```python
from build123d import *

# Parameters (mm, degrees)
SKETCH_R          = 5
PAD_DEPTH         = 5
POCKET_DEPTH      = 25.001
POCKET_DEPTH_BACK = 25.001


with BuildPart() as part:
    # Sketch → Pad (new body)
    with BuildSketch(Plane.XY):
        with BuildLine():
            Line((-50, 15), (-50, -15))
            ThreePointArc((-50, -15), (-47.071068, -22.071068), (-40, -25))
            Line((-40, -25), (0, -25))
            Line((0, -25), (0, 25))
            Line((0, 25), (-40, 25))
            ThreePointArc((-40, 25), (-47.071068, 22.071068), (-50, 15))
        make_face()
        with Locations((-40, 15)):
            Circle(SKETCH_R, mode=Mode.SUBTRACT)
        with Locations((-40, -15)):
            Circle(SKETCH_R, mode=Mode.SUBTRACT)
    extrude(amount=PAD_DEPTH)

    # Sketch001 → Pocket (cut, two sides)
    with BuildSketch(Plane.XZ) as pocket_sk:
        Polygon((0, 3), (-24, 3), (-24.890457, 5), (0, 5), align=None)
    extrude(amount=-POCKET_DEPTH, mode=Mode.SUBTRACT)
    extrude(pocket_sk.sketch, amount=POCKET_DEPTH_BACK, mode=Mode.SUBTRACT)

    # Mirrored: part across YZ


with BuildPart() as part_1:
    add(part.part)
    add(part.part.mirror(Plane.YZ))


solid = part_1.part
```
Verification items for the finished model (mm, model axes). A direction names the side the tool comes from. Round coordinates to 2 decimals unless told otherwise and drop trailing zeros. Order: outer loops, then holes, each group sorted by start corner. A loop starts at its lowest first (then second) coordinate and runs counter-clockwise, first axis right, second up.
1) Cross-section at D-D, the plane y = -8.5. Record the cut outline in (x, z).
Geometry says:
outline: (-50, 0) - (50, 0) - (50, 5) - (24.89, 5) - (24, 3) - (-24, 3) - (-24.89, 5) - (-50, 5) - close
2) Material ranges on line 1 (Y direction, x = -40, z = 4); line 2 (X direction, y = 13.5, z = 4.05); line 3 (Y direction, x = 38.5, z = 4.85), recorded low to high.
Geometry says:
line 1: y = -25 to -20, -10 to 10, 20 to 25
line 2: x = -50 to -44.77, -35.23 to -24.47, 24.47 to 35.23, 44.77 to 50
line 3: y = -25 to -19.77, -10.23 to 10.23, 19.77 to 25
3) Depth check by flat-ended pin: pin 1 (2 mm diameter, centred on y = 17.5, z = 2.5, fed in from +X); pin 2 (1.5 mm diameter, centred on x = -4, y = -14.5, fed in from +Z); pin 3 (1 mm diameter, centred on x = 36.5, y = 14, fed in from +Z). Enter the tip coordinate at first touch or a pass-through.
Geometry says:
pin 1: stops at x = 49.89
pin 2: stops at z = 3
pin 3: passes through
4) Tool access check on faces 4 (the flat face through (0, 0, 3)), 5 (the cylindrical face through (47.15, -21.99, 2.46)). Record the directions out of +Z, -Z, +X, -X, +Y, -Y that give a thin tool (end or side, any length) a straight path to the whole face; none if there is none.
Geometry says:
face 4: +Z, +Y, -Y
face 5: +Z, -Z, +X, -Y
5) Cross-section at B-B, the plane y = 17.5. Record the cut outline in (x, z).
Geometry says:
outline: (-49.68, 0) - (-44.33, 0) - (-44.33, 5) - (-49.68, 5) - close; (-35.67, 0) - (35.67, 0) - (35.67, 5) - (24.89, 5) - (24, 3) - (-24, 3) - (-24.89, 5) - (-35.67, 5) - close; (44.33, 0) - (49.68, 0) - (49.68, 5) - (44.33, 5) - close
6) Cross-section at A-A, the plane x = -36. Record the cut outline in (y, z), plus the area to 3 significant figures.
Geometry says:
outline: (-25, 0) - (-18, 0) - (-18, 5) - (-25, 5) - close; (-12, 0) - (12, 0) - (12, 5) - (-12, 5) - close; (18, 0) - (25, 0) - (25, 5) - (18, 5) - close
area: 190 mm2
7) Cross-section at C-C, the plane z = 3.9. Record the cut outline in (x, y), plus the area to 3 significant figures.
Geometry says:
outline: (-50, -15) arc R10 ccw to (-40, -25) - (-24.4, -25) - (-24.4, 25) - (-40, 25) arc R10 ccw to (-50, 15) - close; (24.4, -25) - (40, -25) arc R10 ccw to (50, -15) - (50, 15) arc R10 ccw to (40, 25) - (24.4, 25) - close; hole circle Ø10 at (-40, -15); hole circle Ø10 at (-40, 15); hole circle Ø10 at (40, -15); hole circle Ø10 at (40, 15)
area: 2,160 mm2
8) Draft check along Y on faces 1 (the cylindrical face through (44, 12, 2)), 2 (the flat face through (-24.44, -0.35, 3.99)), 3 (the flat face through (1, -25, 2)). Enter one of: +Y half, -Y half, draft (parallel to the pull), parting line (faces both ways), or undercut.
Geometry says:
face 1: undercut
face 2: draft
face 3: -Y half
